Could you check a few things on this model? Use its own coordinates, in mm. A direction names the side the tool comes from. Coordinates: 2 decimals unless noted, no trailing zeros. Loops run counter-clockwise (first coordinate to the right, second up) from the corner with the lowest first, then second, coordinate; pieces in that order, holes last. Notation, with made-up numbers: M 9,21 L 17,21 A20 cw 17,59 Z; hole C 48.25,44.5 d8. An arc over 180 degrees is marked long. Write each question's results on one line, items separated by ' | '.
```python
from build123d import *

# Parameters (mm, degrees)
SKETCH1_R           = 76.2
BOSS_EXTRUDE1_DEPTH = 129.54
CUT_EXTRUDE1_START  = -5.08
SKETCH2_R           = 76.2
SKETCH2_W           = 62.08
SKETCH2_H           = 62.08
CUT_EXTRUDE1_DEPTH  = 119.38
SKETCH3_W           = 57
SKETCH3_H           = 57
CUT_EXTRUDE2_DEPTH  = 129.54
SKETCH4_R           = 2.0828
CUT_EXTRUDE3_DEPTH  = 5.08
SKETCH5_R           = 12.7
CUT_EXTRUDE4_DEPTH  = 5.08
SKETCH8_W           = 14
SKETCH8_H           = 5
CUT_EXTRUDE5_DEPTH  = 169.503684233
SKETCH9_W           = 19.05
SKETCH9_H           = 7.62
CUT_EXTRUDE6_DEPTH  = 15.24


with BuildPart() as part:
    # Sketch1 → Boss-Extrude1 (new body)
    with BuildSketch(Plane.XY):
        Circle(SKETCH1_R)
    extrude(amount=BOSS_EXTRUDE1_DEPTH)

    # Sketch2 → Cut-Extrude1 (cut)
    with BuildSketch(Plane(origin=(0, 0, 0), x_dir=(-1, 0, 0), z_dir=(0, 0, -1)).offset(CUT_EXTRUDE1_START)):
        Circle(SKETCH2_R)
        Rectangle(SKETCH2_W, SKETCH2_H, mode=Mode.SUBTRACT)
    extrude(amount=-CUT_EXTRUDE1_DEPTH, mode=Mode.SUBTRACT)

    # Sketch3 → Cut-Extrude2 (cut)
    with BuildSketch(Plane(origin=(0, 0, 0), x_dir=(-1, 0, 0), z_dir=(0, 0, -1))):
        Rectangle(SKETCH3_W, SKETCH3_H)
    extrude(amount=-CUT_EXTRUDE2_DEPTH, mode=Mode.SUBTRACT)

    # Sketch4 → Cut-Extrude3 (cut)
    with BuildSketch(Plane(origin=(0, 0, 0), x_dir=(-1, 0, 0), z_dir=(0, 0, -1))):
        with Locations((0, 63.5)):
            Circle(SKETCH4_R)
        with Locations((54.99261314, -31.75)):
            Circle(SKETCH4_R)
        with Locations((-54.99261314, -31.75)):
            Circle(SKETCH4_R)
    extrude(amount=-CUT_EXTRUDE3_DEPTH, mode=Mode.SUBTRACT)

    # Sketch5 → Cut-Extrude4 (cut)
    with BuildSketch(Plane.XY.offset(129.54)):
        with Locations((0, 57.15)):
            Circle(SKETCH5_R)
        with Locations((49.493351826, -28.575)):
            Circle(SKETCH5_R)
        with Locations((-49.493351826, -28.575)):
            Circle(SKETCH5_R)
    extrude(amount=-CUT_EXTRUDE4_DEPTH, mode=Mode.SUBTRACT)

    # Sketch8 → Cut-Extrude5 (cut, through all)
    with BuildSketch(Plane.XY.offset(129.54)):
        with Locations((0, -31)):
            Rectangle(SKETCH8_W, SKETCH8_H)
    extrude(amount=-CUT_EXTRUDE5_DEPTH, mode=Mode.SUBTRACT)

    # Sketch9 → Cut-Extrude6 (cut)
    with BuildSketch(Plane(origin=(0, 0, 0), x_dir=(-1, 0, 0), z_dir=(0, 0, -1))):
        with Locations((0, 28.5)):
            Rectangle(SKETCH9_W, SKETCH9_H)
    extrude(amount=-CUT_EXTRUDE6_DEPTH, mode=Mode.SUBTRACT)


solid = part.part
```
(1) Will these pins go through, and if not, where does the flat tip stop? P1, Ø3, axis at x = -24.5, z = 49.5, coming from the -Y side; P2, Ø5.5, axis at y = -30.5, z = 65.5, coming from the -X side; P3, Ø4, axis at x = -3.5, z = 1.5, coming from the +Y side; P4, Ø5.5, axis at x = 0, y = 63.5, coming from the -Z side.
Reported:
P1: stops at y = -31.04 | P2: stops at x = -31.04 | P3: stops at y = 76.19 | P4: stops at z = 0
(2) Please list where these lines run through material, in increasing order: probe 1 along Z at (x, y) = (-34.5, 61.5); probe 2 along X at (y, z) = (-4.5, 115). Write a range as from..to.
Reported:
probe 1: z = 0..5.08, 124.46..129.54 | probe 2: x = -31.04..-28.5, 28.5..31.04
(3) Imagine slicing it at D-D, the plane y = 57.15. List the corners of the cut face in (x, z) for me, and give its area (3 significant figures).
Reported:
outline: M -50.4,0 L 50.4,0 L 50.4,5.08 L -50.4,5.08 Z; M -50.4,124.46 L -12.7,124.46 L -12.7,129.54 L -50.4,129.54 Z; M 12.7,124.46 L 50.4,124.46 L 50.4,129.54 L 12.7,129.54 Z | area: 895 mm2
(4) Imagine slicing it at A-A, the plane z = 12. List the corners of the cut face in (x, y) for me (3 decimals).
Reported:
outline: M -31.04,-31.04 L -7,-31.04 L -7,-28.5 L -28.5,-28.5 L -28.5,28.5 L -9.525,28.5 L -9.525,31.04 L -31.04,31.04 Z; M 7,-31.04 L 31.04,-31.04 L 31.04,31.04 L 9.525,31.04 L 9.525,28.5 L 28.5,28.5 L 28.5,-28.5 L 7,-28.5 Z
(5) If we mould it in two halves opening along Z, with no side actions, what happens to faces 6 (the flat face through (19, -31.04, 64)), 7 (the cylindrical face through (-56.917, -32.548, 2.504)), 8 (the flat face through (33, 1, 0)), 9 (the flat face through (31.04, 0, 64))? For each: released by +Z, released by -Z, zero draft, split by the parting line, or undercut.
Reported:
face 6: undercut | face 7: zero draft | face 8: released by -Z | face 9: undercut
(6) Imagine slicing it at C-C, the plane y = 0. List the corners of the cut face in (x, z) for me.
Reported:
outline: M -76.2,0 L -28.5,0 L -28.5,129.54 L -76.2,129.54 L -76.2,124.46 L -31.04,124.46 L -31.04,5.08 L -76.2,5.08 Z; M 28.5,0 L 76.2,0 L 76.2,5.08 L 31.04,5.08 L 31.04,124.46 L 76.2,124.46 L 76.2,129.54 L 28.5,129.54 Z
(7) Which directions (+Z, -Z, +X, -X, +Y, -Y) give clear straight access to the entire face, cutting with the end or side of a thin tool? Please do faces 1 (the flat face through (-31.04, 0, 64)), 2 (the flat face through (-28.5, 0, 64)), 3 (the flat face through (0, 31.04, 64)), 4 (the cylindrical face through (47.84, -15.983, 127.036)), 5 (the flat face through (-9.525, 30, 8)).
Reported:
face 1: -X, +Y, -Y | face 2: +Z, -Z | face 3: +X, -X, +Y | face 4: +Z | face 5: -Z
(8) Imagine slicing it at B-B, the plane x = 0. List the corners of the cut face in (y, z) for me.
Reported:
outline: M -76.2,0 L -33.5,0 L -33.5,5.08 L -76.2,5.08 Z; M -76.2,124.46 L -33.5,124.46 L -33.5,129.54 L -76.2,129.54 Z; M 28.5,15.24 L 31.04,15.24 L 31.04,124.46 L 44.45,124.46 L 44.45,129.54 L 28.5,129.54 Z; M 32.31,0 L 61.42,0 L 61.42,5.08 L 32.31,5.08 Z; M 65.58,0 L 76.2,0 L 76.2,5.08 L 65.58,5.08 Z; M 69.85,124.46 L 76.2,124.46 L 76.2,129.54 L 69.85,129.54 Z
